Could you check a few things on this model? Use its own coordinates, in mm. A direction names the side the tool comes from. Give positions to 0.01 mm unless a question says otherwise; leave off trailing zeros. Order: outer loops, then holes, each group sorted by start corner. A loop starts at its lowest first (then second) coordinate and runs counter-clockwise, first axis right, second up. Notation, with made-up numbers: (48, -38) - (63, -38) arc R15 ccw to (63, -19) - close; hole circle Ø9 at (-22, 86). An arc over 180 degrees is marked (long way). One line per question, with ' | ' between items. Start each with the question number.
1. If we mould it in two halves opening along Z, with no side actions, what happens to faces 1 (the flat face through (1, 20, -33)), 2 (the cylindrical face through (-5.305, 3.757, 120.533)), 3 (the cylindrical face through (-32.761, 9.86, 51.436))? For each: released by +Z, released by -Z, zero draft, split by the parting line, or undercut.
2. Imagine slicing it at D-D (x = 97.5). Please give me the cut outline in (y, z), and give its area (3 significant figures).
3. Which directions (+Z, -Z, +X, -X, +Y, -Y) give clear straight access to the entire face, cutting with the end or side of a thin tool? Please do faces 4 (the cylindrical face through (51.436, 9.86, 32.761)), 5 (the cylindrical face through (-15.456, 13.723, 20.157)), 6 (the flat face through (0, 1.016, 0)).
4. For P1, Ø10, axis at x = -71, z = 45.5, coming from the +Y side; P2, Ø3, axis at y = 2.5, z = -50.5, coming from the -X side; P3, Ø8, axis at x = -45.5, y = 7, coming from the +Z side, each with a flat end and sliding along its axis, tell me the tip position at first contact or that it passes through.
5. Imagine slicing it at A-A (y = 10.5). Give the number of separate pieces and of enclosed holes in the cut face, and give its area (3 significant figures).
6. I need wall thicknesses on probe 1 along Z at (x, y) = (16.5, 11.25); probe 2 along X at (y, z) = (13.5, -8); probe 3 along Z at (x, y) = (61, 17.75). Which ranges of each line are inside material? Lowest first, please. Write a range as from..to.
7. Imagine slicing it at B-B (x = 0). Please give me the cut outline in (y, z).
8. Imagine slicing it at C-C (z = -0.5). Please give me the cut outline in (x, y).
```python
from build123d import *

# Parameters (mm, degrees)
SKETCH1_R         = 120.65
EXTRUDE1_DEPTH    = 7.62
SKETCH2_R         = 76.0000004
SKETCH2_R_2       = 25.4
EXTRUDE2_DEPTH    = 20
EXTRUDE3_DEPTH    = 1.016
EXTRUDE4_REACH    = 173.793
SKETCH8_R         = 4.2
CIRPATTERN1_COUNT = 16


with BuildPart() as part:
    # Sketch1 → Extrude1 (new body)
    with BuildSketch(Plane(origin=(0, 0, 0), x_dir=(1, 0, 0), z_dir=(0, 1, 0))):
        with Locations(Location((0, 0, 0), (0, 0, 90))):
            Circle(SKETCH1_R)
    extrude(amount=EXTRUDE1_DEPTH)

    # Sketch2 → Extrude2 (add)
    with BuildSketch(Plane.XZ):
        with Locations(Location((0, 0, 0), (0, 0, 270))):
            Circle(SKETCH2_R)
        with Locations(Location((0, 0, 0), (0, 0, 270))):
            Circle(SKETCH2_R_2, mode=Mode.SUBTRACT)
    extrude(amount=-EXTRUDE2_DEPTH)

    # Sketch5 → Extrude3 (cut)
    with BuildSketch(Plane.XZ):
        Polygon((28.869265873, -70.307862916), (27.394526953, -70.895486407), (-28.869265873, 70.307862916), (-27.394526953, 70.895486407), align=None)
    extrude(amount=-EXTRUDE3_DEPTH, mode=Mode.SUBTRACT)

    # Sketch8 → Extrude4 (cut, up to next)
    with BuildSketch(Plane.XZ, mode=Mode.PRIVATE) as extrude4_sk1:
        with Locations(Location((-11.84499556, 64.064175482, 0), (0, 0, 270))):
            Circle(SKETCH8_R)
    extrude4_tool1 = extrude(extrude4_sk1.sketch, amount=-EXTRUDE4_REACH, mode=Mode.PRIVATE) & part.part
    extrude4 = extrude4_tool1.solids().sort_by_distance((-11.844996, 0, 64.064175))[0]
    add(extrude4, mode=Mode.SUBTRACT)

    # CirPattern1: Extrude4 ×16 about axis
    cirpattern1_axis = Axis((0, 0, 0), (0, 1, 0))
    for i in range(1, CIRPATTERN1_COUNT):
        add(extrude4.rotate(cirpattern1_axis, i * 360 / CIRPATTERN1_COUNT), mode=Mode.SUBTRACT)


solid = part.part
```
Results found:
1) face 1: zero draft | face 2: split by the parting line | face 3: undercut
2) outline: (0, -71.06) - (7.62, -71.06) - (7.62, 71.06) - (0, 71.06) - close | area: 1,080 mm2
3) face 4: +Y, -Y | face 5: +Y | face 6: -Y
4) P1: stops at y = 7.62 | P2: stops at x = -110.25 | P3: stops at z = 113.29
5) separate pieces: 1 | enclosed holes: 17 | area: 15,200 mm2
6) probe 1: z = -74.19..-19.31, 19.31..60.71, 66.73..74.19 | probe 2: x = -75.58..-65.75, -62.37..-24.11, 24.11..75.58 | probe 3: z = -45.33..-16.77, -10.37..8.97, 14.72..45.33
7) outline: (0, -120.65) - (7.62, -120.65) - (7.62, -76) - (20, -76) - (20, -25.4) - (7.62, -25.4) - (7.62, 25.4) - (20, 25.4) - (20, 76) - (7.62, 76) - (7.62, 120.65) - (0, 120.65) - (0, 2.14) - (1.02, 2.14) - (1.02, -2.14) - (0, -2.14) - close
8) outline: (-120.65, 0) - (-0.66, 0) - (-0.66, 1.02) - (1.05, 1.02) - (1.05, 0) - (120.65, 0) - (120.65, 7.62) - (76, 7.62) - (76, 20) - (25.4, 20) - (25.4, 7.62) - (-25.4, 7.62) - (-25.4, 20) - (-76, 20) - (-76, 7.62) - (-120.65, 7.62) - close
